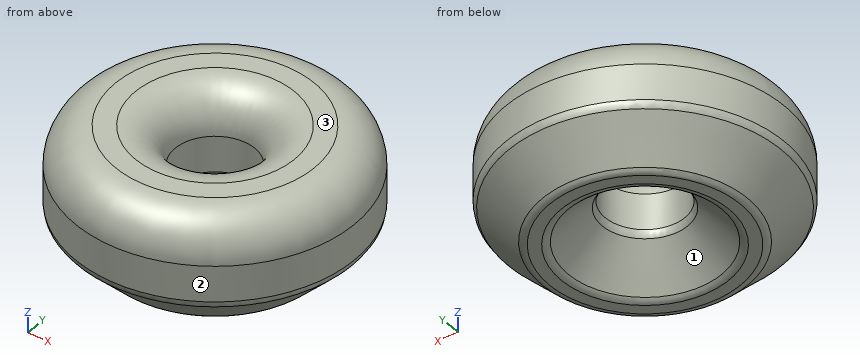
```python
from build123d import *

# Parameters (mm, degrees)
F0_R     = 70
F0_R_2   = 20
F1_DEPTH = 60
F2_R     = 20
F3_SIZE  = 20
F4_R     = 20
F5_R     = 5


with BuildPart() as f1:
    # F0 (on Top) → F1 (new body)
    with BuildSketch(Plane.XY):
        Circle(F0_R)
        Circle(F0_R_2, mode=Mode.SUBTRACT)
    extrude(amount=F1_DEPTH)

    # F2
    f2_edges = [f1.edges().sort_by_distance(p)[0] for p in [
        (-70, 0, 60),
    ]]
    fillet(f2_edges, radius=F2_R)

    # F3
    f3_edges = [f1.edges().sort_by_distance(p)[0] for p in [
        (-70, 0, 0),
        (-20, 0, 0),
    ]]
    chamfer(f3_edges, length=F3_SIZE)

    # F4
    f4_edges = [f1.edges().sort_by_distance(p)[0] for p in [
        (-20, 0, 60),
    ]]
    fillet(f4_edges, radius=F4_R)

    # F5
    f5_edges = [f1.edges().sort_by_distance(p)[0] for p in [
        (-70, 0, 20),
        (-50, 0, 0),
        (-40, 0, 0),
        (-20, 0, 20),
    ]]
    fillet(f5_edges, radius=F5_R)


solid = f1.part
```
For this review, take the finished solid that the model builds, in its own axes (mm). Face numbers are marked on the shaded views. Coordinates: 2 decimals unless noted, no trailing zeros. Write each loop counter-clockwise with the first axis right and the second up, starting at its lowest first coordinate (ties: lowest second). Pieces come first, ordered by that corner, then holes.
(1) For pin 1 Ø1 at (x, z) = (-8.5, 32) entering from -Y; pin 2 Ø8 at (x, z) = (-16.5, 13) entering from -Y; pin 3 Ø5 at (x, z) = (-44.5, 41.5) entering from -Y, all flat-tipped, find the tip position at first contact; note any pin that passes through.
(2) Wall thickness on probe 1 along Y at (x, z) = (0, 32.75); probe 2 along X at (y, z) = (-12, 47): over which ranges is each line inside the solid? List them lowest first.
(3) Add section A-A on z = 12. Give the boundary of the cut face in (x, y).
(4) The part is to be moulded in two halves that separate along Y. For the marked faces 1, 2 and 3, say which applies: +Y half, -Y half, draft (parallel to the pull), parting line (faces both ways), or undercut.
(5) Add section B-B on z = 35. Give the boundary of the cut face in (x, y).
Answer sheet:
1. pin 1: stops at y = -69.54
1. pin 2: stops at y = -65.05
1. pin 3: stops at y = -55.94
2. probe 1: y = -70 to -20, 20 to 70
2. probe 2: x = -67.68 to -17.56, 17.56 to 67.68
3. outline: circle Ø124 at (0, 0); hole circle Ø56 at (0, 0)
4. face 1: undercut
4. face 2: parting line
4. face 3: draft
5. outline: circle Ø140 at (0, 0); hole circle Ø40 at (0, 0)
